```python
from build123d import *

# Parameters (mm, degrees)
BOSS_EXTRU_1_DEPTH = 3
BOSS_EXTRU_2_DEPTH = 1.5


# Read off the part's stored shape, not the designer's step: Boss.-Extru.1
with BuildPart() as part:
    # Boss.-Extru.1 outline → Boss.-Extru.1 (new body)
    with BuildSketch(Plane.XY):
        with BuildLine():
            Line((-2.42213609, 2.526510788), (-2.068537469, 14))
            ThreePointArc((-2.068537469, 14), (-1.893416293, 14.818423654), (-1.398720191, 15.493523995))
            ThreePointArc((-1.398720191, 15.493523995), (-0.093015019, 18.999976034), (1.246958654, 15.506476005))
            ThreePointArc((1.246958654, 15.506476005), (1.752312916, 14.827347495), (1.931462531, 14))
            Line((1.931462531, 14), (2.396407287, 2.550927696))
            ThreePointArc((2.396407287, 2.550927696), (3.208864051, 1.397566279), (3.49995806, 0.017134162))
            Line((3.49995806, 0.017134162), (3.508676576, 0.017176844))
            Line((3.508676576, 0.017176844), (3.425452507, 17.017176844))
            ThreePointArc((3.425452507, 17.017176844), (-0.100400913, 20.508676576), (-3.591900645, 16.982823156))
            Line((-3.591900645, 16.982823156), (-3.508676576, -0.017176844))
            Line((-3.508676576, -0.017176844), (-3.49995806, -0.017134162))
            ThreePointArc((-3.49995806, -0.017134162), (-3.222628149, 1.3655284), (-2.42213609, 2.526510788))
        make_face()
    extrude(amount=BOSS_EXTRU_1_DEPTH)

    # Esquisse1<5> → Boss.-Extru.2 (add)
    with BuildSketch(Plane.XY):
        with BuildLine():
            ThreePointArc((-2.065775424, 14.105074011), (-2.067846838, 14.052555154), (-2.068537469, 14))
            Line((-2.068537469, 14), (-1.902868639, 14))
            ThreePointArc((-1.902868639, 14), (-1.985047825, 14.051411734), (-2.065775424, 14.105074011))
        make_face()
        with BuildLine():
            Line((-1.902868639, 14), (-2.068537469, 14))
            ThreePointArc((-2.068537469, 14), (-0.068537469, 12), (1.931462531, 14))
            Line((1.931462531, 14), (1.7364205, 14))
            ThreePointArc((1.7364205, 14), (-0.083224069, 13.491281379), (-1.902868639, 14))
        make_face()
        with BuildLine():
            Line((1.7364205, 14), (1.931462531, 14))
            ThreePointArc((1.931462531, 14), (1.930490661, 14.062342092), (1.927575995, 14.124623596))
            ThreePointArc((1.927575995, 14.124623596), (1.833011637, 14.060757397), (1.7364205, 14))
        make_face()
        with BuildLine():
            ThreePointArc((-2.065775424, 14.105074011), (-1.985047825, 14.051411734), (-1.902868639, 14))
            Line((-1.902868639, 14), (1.7364205, 14))
            ThreePointArc((1.7364205, 14), (1.833011637, 14.060757397), (1.927575995, 14.124623596))
            ThreePointArc((1.927575995, 14.124623596), (1.725638814, 14.88370327), (1.246958654, 15.506476005))
            ThreePointArc((1.246958654, 15.506476005), (-0.073433119, 15.000023966), (-1.398720191, 15.493523995))
            ThreePointArc((-1.398720191, 15.493523995), (-1.871279944, 14.866094433), (-2.065775424, 14.105074011))
        make_face()
        with BuildLine():
            Line((1.7364205, 14), (-1.902868639, 14))
            ThreePointArc((-1.902868639, 14), (-0.083224069, 13.491281379), (1.7364205, 14))
        make_face()
        with BuildLine():
            Line((-2.068537469, 14), (-2.42213609, 2.526510788))
            ThreePointArc((-2.42213609, 2.526510788), (-0.017735252, 3.499955066), (2.396407287, 2.550927696))
            Line((2.396407287, 2.550927696), (1.931462531, 14))
            ThreePointArc((1.931462531, 14), (-0.068537469, 12), (-2.068537469, 14))
        make_face()
    extrude(amount=BOSS_EXTRU_2_DEPTH)


solid = part.part
```
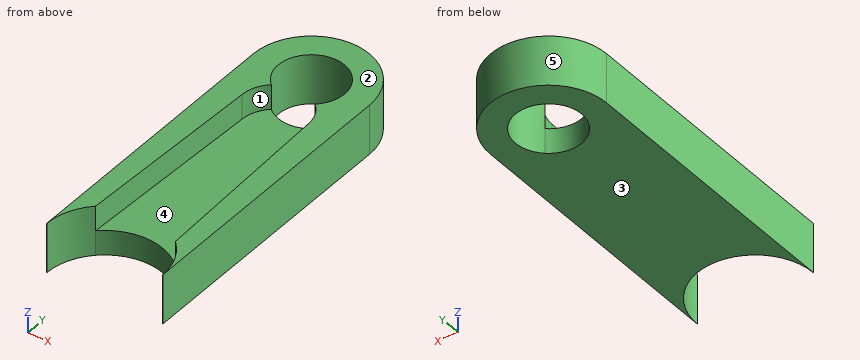
Design review of the part built by this model. Coordinates are the model's own, in mm. Face numbers are marked on the shaded views. A direction names the side the tool comes from. Give positions to 0.01 mm unless a question says otherwise; leave off trailing zeros. Write each loop counter-clockwise with the first axis right and the second up, starting at its lowest first coordinate (ties: lowest second). Pieces come first, ordered by that corner, then holes. Notation, with made-up numbers: (15, 49.25) - (70, 49.25) arc R5 ccw to (70, 55.25) - close; hole circle Ø11 at (47, 39.25). An arc over 180 degrees is marked (long way). Return JSON: item names as keys, results as strings. Group by question number.
(1) Insertion check: pin 1 (1 mm diameter, centred on y = 17.5, z = 2.5, fed in from +X); pin 2 (2.5 mm diameter, centred on x = -0.08, y = 17, fed in from -Z); pin 3 (1 mm diameter, centred on y = 12, z = 1.5, fed in from +X); pin 4 (4 mm diameter, centred on x = 0, y = 10.5, fed in from +Z). Each pin has a flat end and moves straight along its axis. Give the tip position at first contact, or say it passes through.
(2) To check wall thickness, follow probe 1 along X at (y, z) = (17, 1.95); probe 2 along Y at (x, z) = (0, 0.6); probe 3 along Z at (x, y) = (-0.75, 6.75). State the ranges of each line that lie inside material, in increasing order.
(3) Mouldability with a two-part tool opening along X and no side actions: class the marked faces 3, 4 and 5 as +X half, -X half, draft (parallel to the pull), parting line (faces both ways), or undercut.
(4) We need section D-D, the plane y = 12. Give the boundary of the cut face in (x, z), then the cut area to 3 significant figures.
(5) We need section B-B, the plane y = 18.25. Give the boundary of the cut face in (x, z), then the cut area to 3 significant figures.
(6) Machinability: for the marked faces 1 and 2, which of the approach directions +Z, -Z, +X, -X, +Y, -Y give a long, thin tool a straight path to every point of the face, cutting with its end or side? Answer none if there is none.
Reported:
{
 "1": {"pin 1": "stops at x = 3.43", "pin 2": "passes through", "pin 3": "stops at x = 3.45", "pin 4": "stops at z = 1.5"},
 "2": {"probe 1": "x = -3.59 to -2.08, 1.92 to 3.43", "probe 2": "y = 3.5 to 15, 19 to 20.51", "probe 3": "z = 0 to 1.5"},
 "3": {"face 3": "draft", "face 4": "undercut", "face 5": "parting line"},
 "4": {"outline": "(-3.57, 0) - (3.45, 0) - (3.45, 3) - (2.01, 3) - (2.01, 1.5) - (-2.13, 1.5) - (-2.13, 3) - (-3.57, 3) - close", "area": "14.8 mm2"},
 "5": {"outline": "(-3.36, 0) - (-1.64, 0) - (-1.64, 3) - (-3.36, 3) - close; (1.48, 0) - (3.2, 0) - (3.2, 3) - (1.48, 3) - close", "area": "10.3 mm2"},
 "6": {"face 1": "+Z, -Y", "face 2": "+Z, +X, -X, +Y, -Y"}
}
